```python
from build123d import *

# Parameters (mm, degrees)
CROQUIS1_W              = 780
CROQUIS1_H              = 145
CROQUIS1_W_2            = 150
CROQUIS1_H_2            = 5
CROQUIS1_W_3            = 5
CROQUIS1_H_3            = 35
SALIENTE_EXTRUIR1_DEPTH = 5
CORTAR_EXTRUIR1_DEPTH   = 10
CORTAR_EXTRUIR2_DEPTH   = 10


with BuildPart() as part:
    # Croquis1 → Saliente-Extruir1 (new body)
    with BuildSketch(Plane.XY):
        with Locations((390, 72.5)):
            Rectangle(CROQUIS1_W, CROQUIS1_H)
        with Locations((622.5, -2.5)):
            Rectangle(CROQUIS1_W_2, CROQUIS1_H_2)
        Polygon((390, 0), (315, 0), (315, -5), (465, -5), (465, 0), align=None)
        with Locations((157.5, -2.5)):
            Rectangle(CROQUIS1_W_2, CROQUIS1_H_2)
        with Locations((-2.5, 36.25)):
            Rectangle(CROQUIS1_W_3, CROQUIS1_H_3)
        with Locations((782.5, 36.25)):
            Rectangle(CROQUIS1_W_3, CROQUIS1_H_3)
        with Locations((782.5, 108.75)):
            Rectangle(CROQUIS1_W_3, CROQUIS1_H_3)
        with Locations((-2.5, 108.75)):
            Rectangle(CROQUIS1_W_3, CROQUIS1_H_3)
    extrude(amount=SALIENTE_EXTRUIR1_DEPTH)

    # Croquis2 → Cortar-Extruir1 (cut)
    with BuildSketch(Plane.XY.offset(5)):
        Polygon((275.35, 0), (272.15, 0), (272.15, 5), (270.35, 5), (270.35, 8.2), (272.15, 8.2), (272.15, 17.2), (275.35, 17.2), (275.35, 8.2), (277.15, 8.2), (277.15, 5), (275.35, 5), align=None)
        Polygon((507.85, 8.2), (507.85, 17.2), (504.65, 17.2), (504.65, 8.2), (502.85, 8.2), (502.85, 5), (504.65, 5), (504.65, 0), (507.85, 0), (507.85, 5), (509.65, 5), (509.65, 8.2), align=None)
    extrude(amount=-CORTAR_EXTRUIR1_DEPTH, mode=Mode.SUBTRACT)

    # Croquis3 → Cortar-Extruir2 (cut)
    with BuildSketch(Plane.XY.offset(5)):
        Polygon((390, -5), (390, 196.910235404), (-39.994271309, 207.613084807), (-47.647656294, -99.866874564), (0, -99.866874564), align=None)
    extrude(amount=-CORTAR_EXTRUIR2_DEPTH, mode=Mode.SUBTRACT)


solid = part.part
```
Work out the finished part from the listing and answer in its coordinate system (mm). Round coordinates to 2 decimals unless told otherwise and drop trailing zeros. Loops run counter-clockwise (first coordinate to the right, second up) from the corner with the lowest first, then second, coordinate; pieces in that order, holes last.
(1) Each of these flat-tipped pins is pushed along its axis until it touches: P1, Ø2.5, axis at x = 783, z = 1.5, coming from the +Y side; P2, Ø1.4, axis at x = 503.5, z = 3.5, coming from the -Y side; P3, Ø1.5, axis at y = -2, z = 3, coming from the +X side. Where does it stop, or does it pass through?
Computed values:
P1: stops at y = 126.25
P2: stops at y = 0
P3: stops at x = 697.5
(2) The part is cut by section B-B, the plane x = 487. Give the vertices of the cut face in (y, z), and give its area (3 significant figures).
Computed values:
outline: (0, 0) - (145, 0) - (145, 5) - (0, 5) - close
area: 725 mm2
(3) Find the intervals of material crossed by L1, parallel to X at y = 54.5, z = 4.3; L2, parallel to Y at x = 728.5, z = 0.5, in increasing order.
Computed values:
L1: x = 390 to 780
L2: y = 0 to 145
